from build123d import *

# Parameters (mm, degrees)
BOSS_EXTRUDE1_DEPTH      = 0.9
BOSS_EXTRUDE1_DRAFT      = -11
CIRPATTERN1_COPY_1_DEPTH = 0.9
CIRPATTERN1_COPY_1_DRAFT = -11
CIRPATTERN1_COPY_2_DEPTH = 0.9
CIRPATTERN1_COPY_2_DRAFT = -11
CUT_EXTRUDE2_REACH       = 14.838


with BuildPart() as part:
    # Sketch1 → Revolve1 (revolve)
    with BuildSketch(Plane(origin=(0, 0, 0), x_dir=(0, 0, -1), z_dir=(1, 0, 0)), mode=Mode.PRIVATE) as revolve1_sk:
        Polygon((0, 5.8), (2.264331826, 3.9), (2.264331826, 0), (0.5, 0), (0.5, 2.7), (0, 3.6), align=None)
    revolve(revolve1_sk.sketch.rotate(Axis((0, 0, 0), (0, 0, -1)), 90), axis=Axis((0, 0, 0), (0, 0, -1)))


with BuildPart() as boss_extrude1_tool:
    # Sketch7 → Boss-Extrude1 (with draft: the straight prism first)
    with BuildSketch(Plane.XY):
        with BuildLine():
            Line((-2.726795512, 4.280211588), (-2.404415747, 3.77417672))
            ThreePointArc((-2.404415747, 3.77417672), (-1.158215227, 4.322518073), (0.195196758, 4.470740792))
            Line((0.195196758, 4.470740792), (0.221368391, 5.070169725))
            ThreePointArc((0.221368391, 5.070169725), (-1.313506654, 4.902073568), (-2.726795512, 4.280211588))
        make_face()
    extrude(amount=BOSS_EXTRUDE1_DEPTH)
    # Boss-Extrude1: the draft: its side faces are tilted about the plane it starts from
    boss_extrude1_sides = [boss_extrude1_tool.faces().sort_by_distance(p)[0] for p in [
        (0.208282575, 4.770455258, 0.45),
        (-1.313506654, 4.902073568, 0.45),
        (-2.56560563, 4.027194154, 0.45),
        (-1.158215227, 4.322518073, 0.45),
    ]]
    draft(boss_extrude1_sides, Plane.XY, BOSS_EXTRUDE1_DRAFT)


with BuildPart() as part_1:
    add(part.part)

    # Boss-Extrude1: add boss_extrude1_tool
    add(boss_extrude1_tool.part)


with BuildPart() as cirpattern1_copy_1_tool:
    # CirPattern1 copy 1 sketch → CirPattern1 copy 1 (with draft: the straight prism first)
    with BuildSketch(Plane(origin=(0, 0, 0), x_dir=(-0.4999999999999998, 0.8660254037844387, 0), z_dir=(0, 0, 1))):
        with BuildLine():
            Line((-2.726795512, 4.280211588), (-2.404415747, 3.77417672))
            ThreePointArc((-2.404415747, 3.77417672), (-1.158215227, 4.322518073), (0.195196758, 4.470740792))
            Line((0.195196758, 4.470740792), (0.221368391, 5.070169725))
            ThreePointArc((0.221368391, 5.070169725), (-1.313506654, 4.902073568), (-2.726795512, 4.280211588))
        make_face()
    extrude(amount=CIRPATTERN1_COPY_1_DEPTH)
    # CirPattern1 copy 1: the draft: its side faces are tilted about the plane it starts from
    cirpattern1_copy_1_sides = [cirpattern1_copy_1_tool.faces().sort_by_distance(p)[0] for p in [
        (-4.235476729, -2.204849628, 0.45),
        (-3.588566914, -3.588566914, 0.45),
        (-2.204849628, -4.235476729, 0.45),
        (-3.164302846, -3.164302846, 0.45),
    ]]
    draft(cirpattern1_copy_1_sides, Plane(origin=(0, 0, 0), x_dir=(-0.4999999999999998, 0.8660254037844387, 0), z_dir=(0, 0, 1)), CIRPATTERN1_COPY_1_DRAFT)


with BuildPart() as part_2:
    add(part_1.part)

    # CirPattern1 copy 1: add cirpattern1_copy_1_tool
    add(cirpattern1_copy_1_tool.part)


with BuildPart() as cirpattern1_copy_2_tool:
    # CirPattern1 copy 2 sketch → CirPattern1 copy 2 (with draft: the straight prism first)
    with BuildSketch(Plane(origin=(0, 0, 0), x_dir=(-0.5000000000000004, -0.8660254037844384, 0), z_dir=(0, 0, 1))):
        with BuildLine():
            Line((-2.726795512, 4.280211588), (-2.404415747, 3.77417672))
            ThreePointArc((-2.404415747, 3.77417672), (-1.158215227, 4.322518073), (0.195196758, 4.470740792))
            Line((0.195196758, 4.470740792), (0.221368391, 5.070169725))
            ThreePointArc((0.221368391, 5.070169725), (-1.313506654, 4.902073568), (-2.726795512, 4.280211588))
        make_face()
    extrude(amount=CIRPATTERN1_COPY_2_DEPTH)
    # CirPattern1 copy 2: the draft: its side faces are tilted about the plane it starts from
    cirpattern1_copy_2_sides = [cirpattern1_copy_2_tool.faces().sort_by_distance(p)[0] for p in [
        (4.027194154, -2.56560563, 0.45),
        (4.902073568, -1.313506654, 0.45),
        (4.770455258, 0.208282575, 0.45),
        (4.322518073, -1.158215227, 0.45),
    ]]
    draft(cirpattern1_copy_2_sides, Plane(origin=(0, 0, 0), x_dir=(-0.5000000000000004, -0.8660254037844384, 0), z_dir=(0, 0, 1)), CIRPATTERN1_COPY_2_DRAFT)


with BuildPart() as part_3:
    add(part_2.part)

    # CirPattern1 copy 2: add cirpattern1_copy_2_tool
    add(cirpattern1_copy_2_tool.part)

    # Sketch11 → Cut-Extrude2 (cut, up to next)
    with BuildSketch(Plane(origin=(0, -5.298133329, -1.928362829), x_dir=(-1, 0, 0), z_dir=(0, -0.9396926207859081, -0.34202014332566943)), mode=Mode.PRIVATE) as cut_extrude2_sk1:
        with BuildLine():
            Line((0, -0.4), (-2, -0.4))
            ThreePointArc((-2, -0.4), (-2.883883476, -0.766116524), (-3.25, -1.65))
            Line((-3.25, -1.65), (-3.25, -2.9))
            Line((-3.25, -2.9), (-2, -2.9))
            Line((-2, -2.9), (0, -2.9))
            Line((0, -2.9), (1.25, -2.9))
            Line((1.25, -2.9), (1.25, -1.65))
            ThreePointArc((1.25, -1.65), (0.883883476, -0.766116524), (0, -0.4))
        make_face()
    cut_extrude2_tool1 = extrude(cut_extrude2_sk1.sketch, amount=-CUT_EXTRUDE2_REACH, mode=Mode.PRIVATE) & part_3.part
    add(cut_extrude2_tool1.solids().sort_by_distance((1, -5.883514, -0.320042))[0], mode=Mode.SUBTRACT)


solid = part_3.part
Could you check a few things on this model? Use its own coordinates, in mm. A direction names the side the tool comes from. Give positions to 0.01 mm unless a question says otherwise; leave off trailing zeros. Order: outer loops, then holes, each group sorted by start corner. A loop starts at its lowest first (then second) coordinate and runs counter-clockwise, first axis right, second up. Notation, with made-up numbers: (17, 40) -> (69, 40) arc R35 cw to (69, 72) -> close; hole circle Ø9 at (-40, 44.5). An arc over 180 degrees is marked (long way). Return JSON: item names as keys, results as strings.
1. For pin 1 Ø6 at (x, y) = (-1, 0) entering from +Z; pin 2 Ø1 at (x, z) = (1, -1) entering from +Y, each with a flat end and sliding along its axis, tell me the tip position at first contact or that it passes through.
Answer list:
{"pin 1": "stops at z = 0", "pin 2": "stops at y = 5.3"}
2. Imagine slicing it at A-A on z = 0.5. List the corners of the cut face in (x, y) for me.
Answer list:
{"outline": "(-4.63, -2.3) arc R5.17 ccw to (-2.3, -4.63) -> (-1.93, -3.93) arc R4.38 cw to (-3.93, -1.93) -> close; (-2.86, 4.31) -> (-2.43, 3.64) arc R4.38 cw to (0.29, 4.37) -> (0.32, 5.16) arc R5.17 ccw to start; (3.64, -2.43) -> (4.31, -2.86) arc R5.17 ccw to (5.16, 0.32) -> (4.37, 0.29) arc R4.38 cw to start"}
3. I need wall thicknesses on line 1 (Y direction, x = -3, z = -1.05); line 2 (Z direction, x = -1, y = 2.5); line 3 (X direction, y = 1.5, z = -0.15). Which ranges of each line are inside material? Lowest first, please. Write a range as from..to.
Answer list:
{"line 1": "y = -3.9..3.9", "line 2": "z = -2.26..-0.5", "line 3": "x = -5.47..-2.97, 2.97..5.47"}
4. Imagine slicing it at B-B on y = 0. List the corners of the cut face in (x, z) for me (3 decimals).
Answer list:
{"outline": "(-5.8, 0) -> (-3.9, -2.264) -> (3.9, -2.264) -> (5.8, 0) -> (5.075, 0) -> (5.25, 0.9) -> (4.3, 0.9) -> (4.475, 0) -> (3.6, 0) -> (2.7, -0.5) -> (-2.7, -0.5) -> (-3.6, 0) -> close"}
5. On a 3-axis mill with a long thin cutter (end or side, diameter ignored), from which of +Z, -Z, +X, -X, +Y, -Y can I reach the whole of each face in a straight line? I mean faces 1 (the flat face through (4.77, 0.295, 0.444)), 2 (the cylindrical face through (2.7, -3.28, -0.54)), 3 (the flat face through (0.294, 4.757, 0.444)), 4 (the conical face through (-3.09, -3.12, 0.44)). Say none if no direction works.
Answer list:
{"face 1": "-X, +Y", "face 2": "+Z, -Y", "face 3": "+X, -Y", "face 4": "none"}
6. Thinking about a two-plate mould opening in Y: for faces 5 (the flat face through (0.986, -3.459, -0.833)), 6 (the flat face through (0, 0, -0.5)), 7 (the conical face through (-1.31, 4.99, 0.44)), 8 (the flat face through (-2.64, 3.984, 0.444)), which applies, pulls with the +Y half, pulls with the -Y half, needs draft (parallel to the pull), parting line crosses it, or undercut?
Answer list:
{"face 5": "pulls with the -Y half", "face 6": "undercut", "face 7": "pulls with the +Y half", "face 8": "undercut"}
